Geometry: final body of the model. Coordinates: model frame, mm. A direction names the side the tool comes from. Round coordinates to 2 decimals unless told otherwise and drop trailing zeros. Loops run counter-clockwise (first coordinate to the right, second up) from the corner with the lowest first, then second, coordinate; pieces in that order, holes last. Notation, with made-up numbers: (-21.75, 15.5) -> (23.25, 15.5) arc R16 cw to (23.25, 36.5) -> close; hole circle Ø8 at (33.5, -7.5). An arc over 180 degrees is marked (long way). Answer in a Markdown table with one row per item.
```python
from build123d import *

# Parameters (mm, degrees)
SKETCH_R           = 5
PAD_DEPTH          = 10
PAD001_DEPTH       = 10
POLARPATTERN_COUNT = 20
SKETCH002_R        = 2
POCKET_DEPTH       = 7
PAD002_DEPTH       = 1.5
PAD003_DEPTH       = 5.5
SKETCH005_W        = 4
SKETCH005_H        = 1
POCKET001_DEPTH    = 0.5


with BuildPart() as part:
    # Sketch → Pad (new body)
    with BuildSketch(Plane.XY):
        Circle(SKETCH_R)
    extrude(amount=PAD_DEPTH)

    # Sketch001 → Pad001 (join)
    with BuildSketch(Plane.XY):
        with BuildLine():
            ThreePointArc((0.782172, 4.938442), (0.392295, 4.984587), (0, 5))
            ThreePointArc((0, 5), (-0.392295, 4.984587), (-0.782172, 4.938442))
            ThreePointArc((0.782172, 4.938442), (0, 5.784591), (-0.782172, 4.938442))
        make_face()
    pad001 = extrude(amount=PAD001_DEPTH)

    # PolarPattern: Pad001 ×20 about axis
    polarpattern_axis = Axis((0, 0, 0), (0, 0, 1))
    for i in range(1, POLARPATTERN_COUNT):
        add(pad001.rotate(polarpattern_axis, i * 360 / POLARPATTERN_COUNT))

    # Sketch002 (on Face62 of PolarPattern) → Pocket (cut)
    with BuildSketch(Plane.XY.offset(10)):
        Circle(SKETCH002_R)
    extrude(amount=-POCKET_DEPTH, mode=Mode.SUBTRACT)

    # Sketch003 (on Face64 of Pocket) → Pad002 (join)
    with BuildSketch(Plane.XY.offset(3)):
        with BuildLine():
            Line((-1.959592, 0.4), (1.959592, 0.4))
            ThreePointArc((1.959592, -0.4), (2, 0), (1.959592, 0.4))
            Line((1.959592, -0.4), (-1.959592, -0.4))
            ThreePointArc((-1.959592, 0.4), (-2, 0), (-1.959592, -0.4))
        make_face()
    extrude(amount=PAD002_DEPTH)

    # Sketch004 (on Face64 of Pad002) → Pad003 (join)
    with BuildSketch(Plane.XY.offset(4.5)):
        with BuildLine():
            Line((-1.959592, -0.4), (-0.959592, -0.4))
            Line((-0.959592, -0.4), (-0.959592, 0.4))
            Line((-0.959592, 0.4), (-1.959592, 0.4))
            ThreePointArc((-1.959592, 0.4), (-2, 0), (-1.959592, -0.4))
        make_face()
    extrude(amount=PAD003_DEPTH)

    # Sketch005 (on Face1 of Pad003) → Pocket001 (cut)
    with BuildSketch(Plane(origin=(0, 0, 0), x_dir=(1, 0, 0), z_dir=(0, 0, -1))):
        with Locations((-2, 0)):
            Rectangle(SKETCH005_W, SKETCH005_H)
    extrude(amount=-POCKET001_DEPTH, mode=Mode.SUBTRACT)


solid = part.part
```
Item 1: Reachability of faces 1 (the face through (1, 0, 0)), 2 (the face through (-1.3, -0.4, 4.9)) from +Z, -Z, +X, -X, +Y, -Y: full face, straight path, thin tool, end or side. Return the list, or none.
Answer:
| item | result |
|---|---|
| face 1 | -Z, +X, -X, +Y, -Y |
| face 2 | +Z |
Item 2: Cut plane C-C (y = 1.75). Output: boundary loops of the cut face in (x, z).
Answer:
| item | result |
|---|---|
| outline | (-5.51, 0) -> (5.51, 0) -> (5.51, 10) -> (0.97, 10) -> (0.97, 3) -> (-0.97, 3) -> (-0.97, 10) -> (-5.51, 10) -> close |
Item 3: Draft query along Y for faces 3 (the face through (-5.507, -1.77, 4.93)), 4 (the face through (-1.4, 0.1, 10)). Return one class per face: pulls with the +Y half, pulls with the -Y half, needs draft (parallel to the pull), parting line crosses it, or undercut.
Answer:
| item | result |
|---|---|
| face 3 | undercut |
| face 4 | needs draft |
Item 4: Line query: probe 1 along Y at (x, z) = (-1, 6); probe 2 along Y at (x, z) = (-3, 0.75); probe 3 along Y at (x, z) = (4, 5.5). Output: solid intervals per line, ascending. Write a range as [from, to].
Answer:
| item | result |
|---|---|
| probe 1 | y = [-5.32, -1.73], [-0.4, 0.4], [1.73, 5.32] |
| probe 2 | y = [-4.83, 4.83] |
| probe 3 | y = [-3.72, 3.72] |
Item 5: Pin query (flat end, axial travel): pin 1 Ø1 at (y, z) = (1, 3) entering from +X; pin 2 Ø3 at (x, z) = (2.5, 3.5) entering from -Y; pin 3 Ø1 at (x, z) = (1, 1.5) entering from +Y. Return the tip coordinate at first contact, or that it passes through.
Answer:
| item | result |
|---|---|
| pin 1 | stops at x = 5.6 |
| pin 2 | stops at y = -5.54 |
| pin 3 | stops at y = 5.6 |
Item 6: Cut plane D-D (x = -1.5). Output: boundary loops of the cut face in (y, z), then the cut area to 3 significant figures.
Answer:
| item | result |
|---|---|
| outline | (-5.54, 0) -> (-0.5, 0) -> (-0.5, 0.5) -> (0.5, 0.5) -> (0.5, 0) -> (5.54, 0) -> (5.54, 10) -> (1.32, 10) -> (1.32, 3) -> (0.4, 3) -> (0.4, 10) -> (-0.4, 10) -> (-0.4, 3) -> (-1.32, 3) -> (-1.32, 10) -> (-5.54, 10) -> close |
| area | 97.4 mm² |
